Geometry: final body of the model. Coordinates: model frame, mm. Face numbers are marked on the shaded views. A direction names the side the tool comes from. Give positions to 0.01 mm unless a question says otherwise; leave off trailing zeros. Write each loop counter-clockwise with the first axis right and the second up, starting at its lowest first coordinate (ties: lowest second). Pieces come first, ordered by that corner, then holes. Notation, with made-up numbers: (46.5, -17.5) - (79.5, -17.5) arc R28 ccw to (79.5, 10.5) - close; hole circle Ø4 at (74.25, 49.5). An arc over 180 degrees is marked (long way). Return JSON: item names as keys, results as strings.
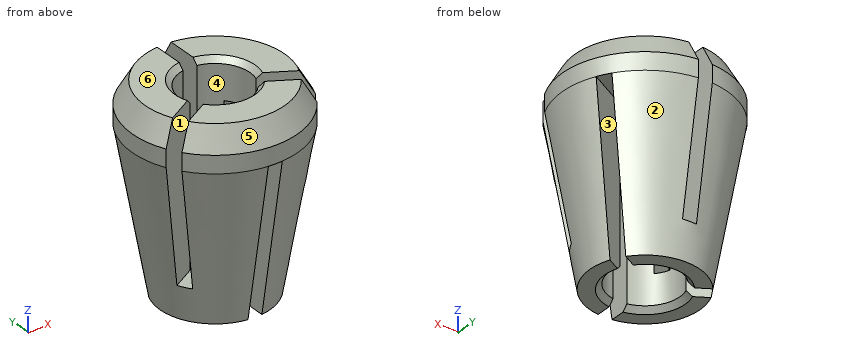
from build123d import *

# Parameters (mm, degrees)
CHAMFER006_SIZE       = 0.3
SKETCH001_W           = 0.8
SKETCH001_H           = 5
POCKET003_DEPTH       = 44.301226966
POLARPATTERN003_COUNT = 3
SKETCH009_W           = 0.8
SKETCH009_H           = 5
POCKET004_DEPTH       = 9
POLARPATTERN004_COUNT = 3


with BuildPart() as part:
    # Sketch008 → Revolution001 (revolve)
    with BuildSketch(Plane.YZ):
        Polygon((-2, 0), (-2, 11.2764224176), (-4, 11.2764224176), (-4.7369428264, 10), (-4.7369428264, 9), (-3.15, 0), align=None)
    revolve(axis=Axis((0, 0, 0), (0, 0, 1)))

    # Chamfer006
    chamfer006_edges = [part.edges().sort_by_distance(p)[0] for p in [
        (0, 2, 11.276422),
        (0, 2, 0),
    ]]
    chamfer(chamfer006_edges, length=CHAMFER006_SIZE)

    # Sketch001 → Pocket003 (cut, through all)
    with BuildSketch(Plane.XY.offset(2)):
        with Locations((0, 2.5)):
            Rectangle(SKETCH001_W, SKETCH001_H)
    pocket003 = extrude(amount=POCKET003_DEPTH, mode=Mode.SUBTRACT)

    # PolarPattern003: Pocket003 ×3 about axis
    polarpattern003_axis = Axis((0, 0, 2), (0, 0, 1))
    for i in range(1, POLARPATTERN003_COUNT):
        add(pocket003.rotate(polarpattern003_axis, i * 360 / POLARPATTERN003_COUNT), mode=Mode.SUBTRACT)

    # Sketch009 → Pocket004 (cut)
    with BuildSketch(Plane.XY):
        with Locations((0, -2.5)):
            Rectangle(SKETCH009_W, SKETCH009_H)
    pocket004 = extrude(amount=POCKET004_DEPTH, mode=Mode.SUBTRACT)

    # PolarPattern004: Pocket004 ×3 about axis
    polarpattern004_axis = Axis((0, 0, 0), (0, 0, 1))
    for i in range(1, POLARPATTERN004_COUNT):
        add(pocket004.rotate(polarpattern004_axis, i * 360 / POLARPATTERN004_COUNT), mode=Mode.SUBTRACT)


with BuildPart() as part_1:
    # Body003 placement: moved
    add(part.part.moved(Location((0, 0, 11.5))))


solid = part_1.part
Q1. Material intervals for probe 1 along X at (y, z) = (0, 19.5); probe 2 along X at (y, z) = (0, 14.75); probe 3 along Z at (x, y) = (-2.75, 1.5), sorted ascending. Write a range as [from, to].
Answer key:
{"probe 1": "x = [-4.56, -2], [2, 4.56]", "probe 2": "x = [-3.72, -2], [2, 3.72]", "probe 3": "z = [20.5, 22.78]"}
Q2. Section query A-A, the plane x = 0. Return the cut outline in (y, z).
Answer key:
{"outline": "(-4.74, 20.5) - (-2, 20.5) - (-2, 22.48) - (-2.3, 22.78) - (-4, 22.78) - (-4.74, 21.5) - close; (2, 11.8) - (2.3, 11.5) - (3.15, 11.5) - (3.5, 13.5) - (2, 13.5) - close"}
Q3. Section query B-B, the plane z = 16.75. Return the cut outline in (x, y), plus the area to 3 significant figures.
Answer key:
{"outline": "(-3.71, -1.68) - (-1.9, -0.63) arc R2 cw to (-1.9, 0.63) - (-3.71, 1.68) arc R4.08 ccw to start; (-3.31, -2.37) arc R4.08 ccw to (-0.4, -4.06) - (-0.4, -1.96) arc R2 cw to (-1.5, -1.33) - close; (-3.31, 2.37) - (-1.5, 1.33) arc R2 cw to (-0.4, 1.96) - (-0.4, 4.06) arc R4.08 ccw to start; (0.4, -4.06) arc R4.08 ccw to (3.31, -2.37) - (1.5, -1.33) arc R2 cw to (0.4, -1.96) - close; (0.4, 1.96) arc R2 cw to (1.5, 1.33) - (3.31, 2.37) arc R4.08 ccw to (0.4, 4.06) - close; (1.9, -0.63) - (3.71, -1.68) arc R4.08 ccw to (3.71, 1.68) - (1.9, 0.63) arc R2 cw to start", "area": "29.6 mm^2"}
Q4. Section query D-D, the plane z = 21. Return the cut outline in (x, y).
Answer key:
{"outline": "(-4.29, -2.01) - (-1.9, -0.63) arc R2 cw to (-0.4, 1.96) - (-0.4, 4.72) arc R4.74 ccw to start; (-3.89, -2.71) arc R4.74 ccw to (3.89, -2.71) - (1.5, -1.33) arc R2 cw to (-1.5, -1.33) - close; (0.4, 1.96) arc R2 cw to (1.9, -0.63) - (4.29, -2.01) arc R4.74 ccw to (0.4, 4.72) - close"}
Q5. Set-up query: the marked faces 1 and 2. Return all of +Z, -Z, +X, -X, +Y, -Y with unobstructed straight access to the full face (end or side cutting, diameter ignored); none if empty.
Answer key:
{"face 1": "+Z", "face 2": "-Z, +Y"}
Q6. Mould query, pull axis Y, two halves, no side actions, for the marked faces 3, 4, 5 and 6. Classes: pulls with the +Y half, pulls with the -Y half, needs draft (parallel to the pull), parting line crosses it, or undercut.
Answer key:
{"face 3": "undercut", "face 4": "undercut", "face 5": "pulls with the -Y half", "face 6": "needs draft"}
Q7. Section query C-C, the plane y = 0. Return the cut outline in (x, z), plus the area to 3 significant figures.
Answer key:
{"outline": "(-4.74, 20.5) - (-3.15, 11.5) - (-2.3, 11.5) - (-2, 11.8) - (-2, 22.48) - (-2.3, 22.78) - (-4, 22.78) - (-4.74, 21.5) - close; (2, 11.8) - (2.3, 11.5) - (3.15, 11.5) - (4.74, 20.5) - (4.74, 21.5) - (4, 22.78) - (2.3, 22.78) - (2, 22.48) - close", "area": "46.3 mm^2"}
Q8. Pin query (flat end, axial travel): P1, Ø1.2, axis at x = -2.5, y = -1.5, coming from the +Z side; P2, Ø1.4, axis at y = 4, z = 16, coming from the +X side; P3, Ø1.4, axis at y = -3.5, z = 17.5, coming from the +X side; P4, Ø3, axis at x = 2, z = 14, coming from the +Y side. Return the tip coordinate at first contact, or that it passes through.
Answer key:
{"P1": "stops at z = 22.78", "P2": "stops at x = 2.18", "P3": "stops at x = 3.16", "P4": "stops at y = 3.66"}
